```python
from build123d import *

# Parameters (mm, degrees)
F1_DEPTH = 38.1
F2_T     = -7.5
F3_W     = 5
F3_H     = 5.5
F3_H_2   = 5.55
F4_DEPTH = 7


with BuildPart() as f1:
    # F0 (on Top) → F1 (new body)
    with BuildSketch(Plane.XY):
        with BuildLine():
            Line((92.5, 63.290403), (-92.5, 63.290403))
            ThreePointArc((-92.5, 63.290403), (-99.571068, 60.361471), (-102.5, 53.290403))
            Line((-102.5, 53.290403), (-102.5, -76.709597))
            ThreePointArc((-102.5, -76.709597), (-99.571068, -83.780664), (-92.5, -86.709597))
            Line((-92.5, -86.709597), (92.5, -86.709597))
            ThreePointArc((92.5, -86.709597), (99.571068, -83.780664), (102.5, -76.709597))
            Line((102.5, -76.709597), (102.5, 53.290403))
            ThreePointArc((102.5, 53.290403), (99.571068, 60.361471), (92.5, 63.290403))
        make_face()
    extrude(amount=F1_DEPTH)

    # F2
    f2_openings = [f1.faces().sort_by_distance(p)[0] for p in [
        (0, -11.709597, 38.1),
    ]]
    offset(amount=F2_T, openings=f2_openings)

    # F3 (on face) → F4 (cut)
    with BuildSketch(Plane.XY.offset(38.1)):
        with Locations((-100, 42.290403)):
            Rectangle(F3_W, F3_H)
        with Locations((-100, 15.290403)):
            Rectangle(F3_W, F3_H)
        with Locations((-100, -11.734597)):
            Rectangle(F3_W, F3_H_2)
        with Locations((-100, -38.709597)):
            Rectangle(F3_W, F3_H)
        with Locations((-100, -65.709597)):
            Rectangle(F3_W, F3_H)
        with Locations((100, -65.709597)):
            Rectangle(F3_W, F3_H)
        with Locations((100, -38.709597)):
            Rectangle(F3_W, F3_H)
        with Locations((100, -11.734597)):
            Rectangle(F3_W, F3_H_2)
        with Locations((100, 15.290403)):
            Rectangle(F3_W, F3_H)
        with Locations((100, 42.290403)):
            Rectangle(F3_W, F3_H)
    extrude(amount=-F4_DEPTH, mode=Mode.SUBTRACT)


solid = f1.part
```
The listing builds one solid part. Answer for the finished solid, in the listing's coordinates (mm). A direction names the side the tool comes from. Give positions to 0.01 mm unless a question says otherwise; leave off trailing zeros. Order: outer loops, then holes, each group sorted by start corner. A loop starts at its lowest first (then second) coordinate and runs counter-clockwise, first axis right, second up.
Item 1: Find the intervals of material crossed by probe 1 along Y at (x, z) = (42, 16.5); probe 2 along X at (y, z) = (-26, 11.5); probe 3 along Z at (x, y) = (-21.5, 33.5), in increasing order.
From the geometry:
probe 1: y = -86.71 to -79.21, 55.79 to 63.29
probe 2: x = -102.5 to -95, 95 to 102.5
probe 3: z = 0 to 7.5
Item 2: The part is cut by section A-A, the plane x = -0.5. Give the vertices of the cut face in (y, z).
From the geometry:
outline: (-86.71, 0) - (63.29, 0) - (63.29, 38.1) - (55.79, 38.1) - (55.79, 7.5) - (-79.21, 7.5) - (-79.21, 38.1) - (-86.71, 38.1) - close
Item 3: For a pull along Y with two mould halves and no side action, classify faces 1 (the face through (1, 63.29, 19)), 2 (the face through (-1, -86.71, 19)), 3 (the face through (-100, -62.96, 35)) as pulls with the +Y half, pulls with the -Y half, needs draft (parallel to the pull), parting line crosses it, or undercut.
From the geometry:
face 1: pulls with the +Y half
face 2: pulls with the -Y half
face 3: undercut
Item 4: The part is cut by section C-C, the plane y = 4. Give the vertices of the cut face in (x, z).
From the geometry:
outline: (-102.5, 0) - (102.5, 0) - (102.5, 38.1) - (95, 38.1) - (95, 7.5) - (-95, 7.5) - (-95, 38.1) - (-102.5, 38.1) - close
Item 5: Which of the six approach directions +Z, -Z, +X, -X, +Y, -Y give full straight-line access (tool end or side, diameter ignored) to faces 4 (the face through (-1, -11, 7.5)), 5 (the face through (-97.5, -12, 35)), 6 (the face through (97.5, -12, 35))?
From the geometry:
face 4: +Z
face 5: +Z, -X
face 6: +Z, +X
Item 6: The part is cut by section B-B, the plane z = 29. Give the vertices of the cut face in (x, y).
From the geometry:
outline: (-102.5, -76.71) arc R10 ccw to (-92.5, -86.71) - (92.5, -86.71) arc R10 ccw to (102.5, -76.71) - (102.5, 53.29) arc R10 ccw to (92.5, 63.29) - (-92.5, 63.29) arc R10 ccw to (-102.5, 53.29) - close; hole (-95, -76.71) arc R2.5 ccw to (-92.5, -79.21) - (92.5, -79.21) arc R2.5 ccw to (95, -76.71) - (95, 53.29) arc R2.5 ccw to (92.5, 55.79) - (-92.5, 55.79) arc R2.5 ccw to (-95, 53.29) - close
Item 7: Given pin 1 Ø4 at (x, y) = (100.5, 41.5) entering from +Z; pin 2 Ø4 at (x, z) = (-100.5, 34) entering from -Y; pin 3 Ø4 at (x, z) = (99, 35) entering from -Y; pin 4 Ø2.5 at (x, z) = (-99.5, 35) entering from +Y, each flat-ended and moving along its own axis, determine where each tip first touches the part or whether it passes through.
From the geometry:
pin 1: stops at z = 38.1
pin 2: stops at y = -84.71
pin 3: stops at y = -85.64
pin 4: stops at y = 61.47
